Autodesk Inventor part; units mm, degrees
ref_plane "YZ Plane" through (0, 0, 0) normal (1, 0, 0) x (0, 1, 0)
ref_plane "XZ Plane" through (0, 0, 0) normal (0, 1, 0) x (-1, 0, 0)
ref_plane "XY Plane" through (0, 0, 0) normal (0, 0, 1) x (1, 0, 0)
sketch "Sketch1" plane through (0, 0, 0) normal (0, 0, 1) x (1, 0, 0)
  line L0 (-146.6185, 70.3133) -> (95.3815, 70.3133)
  line L1 (95.3815, 70.3133) -> (95.3815, -9.6867)
  line L2 (2.9423, -9.6867) -> (-45.2664, -9.6867)
  line L3 (-146.6185, -9.6867) -> (-146.6185, 70.3133)
  line L4 (-116.6185, -9.6867) -> (-45.2664, -9.6867)
  line L5 (65.3815, -9.6867) -> (2.9423, -9.6867)
  arc A0 (-116.6185, -9.6867) -> (-146.6185, -39.6867) centre (-116.6185, -39.6867) ccw
  arc A1 (95.3815, -39.6867) -> (65.3815, -9.6867) centre (65.3815, -39.6867) ccw
  line L6 (-146.6185, -9.6867) -> (-146.6185, -39.6867)
  line L7 (95.3815, -9.6867) -> (95.3815, -39.6867)
  point P0 (0, 0)
  dimension "d0" = 242
  dimension "d1" = 80
  dimension "d2" = 30
extrude "Extrusion1" add sketch "Sketch1" along normal blind 2
sketch "Sketch2" plane through (0, 0, 2) normal (0, 0, 1) x (1, 0, 0)
  line L0 (95.3815, 70.3133) -> (-146.6185, 70.3133)
  line L1 (-146.6185, 70.3133) -> (-114.6185, 70.3133)
  line L2 (-114.6185, 70.3133) -> (-114.6185, 65.3133)
  line L3 (-114.6185, 65.3133) -> (-146.6185, 65.3133)
  line L4 (-146.6185, 65.3133) -> (-146.6185, 70.3133)
  line L5 (-82.6185, 70.3133) -> (-50.6185, 70.3133)
  line L6 (-50.6185, 70.3133) -> (-50.6185, 65.3133)
  line L7 (-50.6185, 65.3133) -> (-82.6185, 65.3133)
  line L8 (-82.6185, 65.3133) -> (-82.6185, 70.3133)
  line L9 (-0.6185, 70.3133) -> (31.3815, 70.3133)
  line L10 (31.3815, 70.3133) -> (31.3815, 65.3133)
  line L11 (31.3815, 65.3133) -> (-0.6185, 65.3133)
  line L12 (-0.6185, 65.3133) -> (-0.6185, 70.3133)
  line L13 (95.3815, -39.6867) -> (95.3815, 70.3133)
  line L14 (95.3815, 70.3133) -> (63.3815, 70.3133)
  line L15 (63.3815, 70.3133) -> (63.3815, 65.3133)
  line L16 (63.3815, 65.3133) -> (95.3815, 65.3133)
  line L17 (95.3815, 65.3133) -> (95.3815, 70.3133)
  point P0 (0, 0)
  dimension "d5" = 32
  dimension "d6" = 32
  dimension "d7" = 32
  dimension "d8" = 32
  dimension "d9" = 32
  dimension "d10" = 32
  dimension "d11" = 50
  dimension "d12" = 5
extrude "Extrusion2" cut sketch "Sketch2" against normal blind 2
sketch "Sketch3" plane through (0, 0, 2) normal (0, 0, 1) x (1, 0, 0)
  line L0 (-146.6185, 65.3133) -> (-146.6185, -39.6867)
  line L1 (-146.6185, 65.3133) -> (-148.6185, 65.3133)
  line L2 (-148.6185, 65.3133) -> (-148.6185, 34.3133)
  line L3 (-148.6185, 34.3133) -> (-146.6185, 34.3133)
  line L4 (-146.6185, 34.3133) -> (-146.6185, 65.3133)
  line L5 (-146.6185, -1.6867) -> (-148.6185, -1.6867)
  line L6 (-148.6185, -1.6867) -> (-148.6185, -37.6867)
  line L7 (-146.6185, -37.6867) -> (-146.6185, -1.6867)
  line L8 (95.3815, -39.6867) -> (95.3815, 65.3133)
  line L9 (95.3815, 65.3133) -> (97.3815, 65.3133)
  line L10 (97.3815, 65.3133) -> (97.3815, 34.3133)
  line L11 (97.3815, 34.3133) -> (95.3815, 34.3133)
  line L12 (95.3815, 34.3133) -> (95.3815, 65.3133)
  line L13 (95.3815, -1.6867) -> (97.3815, -1.6867)
  line L14 (97.3815, -1.6867) -> (97.3815, -37.6867)
  line L15 (95.3815, -37.6867) -> (95.3815, -1.6867)
  line L16 (-148.6185, -37.6867) -> (-146.6185, -37.6867)
  line L17 (95.3815, -39.6867) -> (95.3815, 65.3133)
  line L18 (95.3815, -37.6867) -> (97.3815, -37.6867)
  point P0 (-146.6185, -37.6867)
  point P1 (95.3815, -37.6867)
  dimension "d34" = 31
  dimension "d35" = 36
  dimension "d36" = 2
  dimension "d37" = 2
  dimension "d39" = 36
  dimension "d40" = 36
extrude "Extrusion3" add sketch "Sketch3" against normal blind 2
sketch "Sketch4" plane through (0, 0, 2) normal (0, 0, 1) x (1, 0, 0)
  line L0 (-148.6185, -37.6867) -> (-146.6185, -37.6867)
  line L1 (-148.6185, -37.6867) -> (112.9742, -37.6867)
  line L2 (112.9742, -37.6867) -> (112.9742, -65.6367)
  line L3 (112.9742, -65.6367) -> (-148.6185, -65.6367)
  line L4 (-148.6185, -65.6367) -> (-148.6185, -37.6867)
  point P0 (0, 0)
extrude "Extrusion4" cut sketch "Sketch4" against normal blind 2
properties part number "front"
Design review of the part built by this model. Coordinates are the model's own, in mm. Give positions to 0.01 mm unless a question says otherwise; leave off trailing zeros. Order: outer loops, then holes, each group sorted by start corner. A loop starts at its lowest first (then second) coordinate and runs counter-clockwise, first axis right, second up. Notation, with made-up numbers: M 35,-19 L 81,-19 A8 cw 81,-9 Z; hole C 21.5,33.25 d6. An arc over 180 degrees is marked long. One line per question, with ' | ' between items. Start each with the question number.
Q1. We need section A-A (z = 0.6). Write out the cut boundary in (x, y).
Q2. The part is to be moulded in two halves that separate along X. For faces 1 (the face through (-137.342, -17.995, 0.986)), 2 (the face through (85.64, -17.56, 0.99)), 3 (the face through (-27, 29, 2)), say which applies: +X half, -X half, draft (parallel to the pull), parting line (faces both ways), or undercut.
Q3. We need section B-B (y = 15.5). Write out the cut boundary in (x, z), plus the area to 3 significant figures.
Q4. For L1, parallel to Y at x = -13, z = 1.65; L2, parallel to X at y = 2.5, z = 1.05; L3, parallel to Y at x = 25, z = 0.4, list the stretches that pass through material, from the lowest coordinate up. Write a range as [from, to].
Q5. We need section C-C (x = -90.5). Write out the cut boundary in (y, z).
Q6. For pin 1 Ø1 at (x, z) = (-55, 1.5) entering from -Y; pin 2 Ø0.6 at (y, z) = (67.5, 1) entering from -X; pin 3 Ø1 at (x, z) = (96.5, 1.5) entering from +Y, all flat-tipped, find the tip position at first contact; note any pin that passes through.
Returned:
1) outline: M -148.62,-37.69 L -146.55,-37.69 A30 cw -116.62,-9.69 L 65.38,-9.69 A30 cw 95.31,-37.69 L 97.38,-37.69 L 97.38,-1.69 L 95.38,-1.69 L 95.38,34.31 L 97.38,34.31 L 97.38,65.31 L 63.38,65.31 L 63.38,70.31 L 31.38,70.31 L 31.38,65.31 L -0.62,65.31 L -0.62,70.31 L -50.62,70.31 L -50.62,65.31 L -82.62,65.31 L -82.62,70.31 L -114.62,70.31 L -114.62,65.31 L -148.62,65.31 L -148.62,34.31 L -146.62,34.31 L -146.62,-1.69 L -148.62,-1.69 Z
2) face 1: undercut | face 2: undercut | face 3: draft
3) outline: M -146.62,0 L 95.38,0 L 95.38,2 L -146.62,2 Z | area: 484 mm2
4) L1: [-9.69, 70.31] | L2: [-146.62, 95.38] | L3: [-9.69, 65.31]
5) outline: M -9.69,0 L 70.31,0 L 70.31,2 L -9.69,2 Z
6) pin 1: y = -9.69 | pin 2: x = -114.62 | pin 3: y = 65.31
